The listing builds one solid part. Answer for the finished solid, in the listing's coordinates (mm). A direction names the side the tool comes from. Round coordinates to 2 decimals unless told otherwise and drop trailing zeros. Write each loop counter-clockwise with the first axis right and the second up, starting at its lowest first coordinate (ties: lowest second). Pieces come first, ordered by that corner, then holes. Notation, with made-up numbers: (13, 86) -> (58, 86) arc R21 cw to (58, 125) -> close; hole circle Ø7 at (55.25, 24.5). An arc over 180 degrees is marked (long way). Write each question's results on one line, items separated by ' | '. Start each with the question number.
```python
from build123d import *

# Parameters (mm, degrees)
SKETCH008_R           = 43
SKETCH008_R_2         = 4
PAD002_DEPTH          = 10
SKETCH009_R           = 11
POCKET002_DEPTH       = 7
SKETCH010_R           = 2.5
POCKET003_DEPTH       = 254.066565
POLARPATTERN001_COUNT = 7
SKETCH011_R           = 2.5
POCKET004_DEPTH       = 254.066565
POLARPATTERN002_COUNT = 4


with BuildPart() as sidecap:
    # Sketch008 → Pad002 (new body)
    with BuildSketch(Plane.XZ):
        Circle(SKETCH008_R)
        Circle(SKETCH008_R_2, mode=Mode.SUBTRACT)
    extrude(amount=PAD002_DEPTH)

    # Sketch009 (on Face3 of Pad002) → Pocket002 (cut)
    with BuildSketch(Plane(origin=(0, 0, 0), x_dir=(1, 0, 0), z_dir=(0, 1, 0))):
        Circle(SKETCH009_R)
    extrude(amount=-POCKET002_DEPTH, mode=Mode.SUBTRACT)

    # Sketch010 (on Face3 of Pocket002) → Pocket003 (cut, through all)
    with BuildSketch(Plane.XZ.offset(10)):
        with Locations((0, 15)):
            Circle(SKETCH010_R)
    pocket003 = extrude(amount=-POCKET003_DEPTH, mode=Mode.SUBTRACT)

    # PolarPattern001: Pocket003 ×7 about axis
    polarpattern001_axis = Axis((0, -10, 0), (0, -1, 0))
    for i in range(1, POLARPATTERN001_COUNT):
        add(pocket003.rotate(polarpattern001_axis, i * 360 / POLARPATTERN001_COUNT), mode=Mode.SUBTRACT)

    # Sketch011 (on Face3 of PolarPattern001) → Pocket004 (cut, through all)
    with BuildSketch(Plane.XZ.offset(10)):
        with Locations((0, 37.5)):
            Circle(SKETCH011_R)
    pocket004 = extrude(amount=-POCKET004_DEPTH, mode=Mode.SUBTRACT)

    # PolarPattern002: Pocket004 ×4 about axis
    polarpattern002_axis = Axis((0, -10, 0), (0, -1, 0))
    for i in range(1, POLARPATTERN002_COUNT):
        add(pocket004.rotate(polarpattern002_axis, i * 360 / POLARPATTERN002_COUNT), mode=Mode.SUBTRACT)


with BuildPart() as sidecap_1:
    # Body003 placement: moved
    add(sidecap.part.moved(Location((0, -21, 0))))


with BuildPart() as part_mirroring:
    # Part__Mirroring: instance of SideCap
    add(sidecap_1.part.mirror(Plane(origin=(0, 0, 0), x_dir=(1, 0, 0), z_dir=(0, 1, 0))))


solid = part_mirroring.part
```
Q1. Find the intervals of material crossed by line 1 (Z direction, x = 0, y = 24); line 2 (Z direction, x = 0, y = 29.3); line 3 (X direction, y = 27.5, z = 1), in increasing order.
Q2. Each of these flat-tipped pins is pushed along its axis until it touches: pin 1 (24 mm diameter, centred on x = -1, z = -3, fed in from -Y); pin 2 (2 mm diameter, centred on y = 28, z = 27, fed in from -X); pin 3 (6 mm diameter, centred on x = 29, y = 23.5, fed in from +Z); pin 4 (5 mm diameter, centred on y = 24.5, z = 16.5, fed in from -X). Where does it stop, or does it pass through?
Q3. The part is cut by section D-D, the plane z = -37.5. Write down the section's boundary in (x, y).
Q4. The part is cut by section C-C, the plane y = 23.5. State how many separate pieces and enclosed holes the cut face has, then the cut area to 3 significant figures.
Q5. For faces 1 (the cylindrical face through (-2.38, 24.45, 10.74)), 2 (the cylindrical face through (-35.06, 26.07, -0.54)), determine the directions among +Z, -Z, +X, -X, +Y, -Y from which every point of the face is accessible in a straight line to the end or side of a thin tool.
Q6. The part is cut by section B-B, the plane z = 1.5. Write down the section's boundary in (x, y).
Q7. The part is cut by section A-A, the plane x = 5.5. Write down the section's boundary in (y, z).
Answers follow:
1) line 1: -43 to -40, -35 to -11, 11 to 12.5, 17.5 to 35, 40 to 43 | line 2: -43 to -40, -35 to -4, 4 to 12.5, 17.5 to 35, 40 to 43 | line 3: -42.99 to -39.79, -35.21 to -10.95, 10.95 to 35.21, 39.79 to 42.99
2) pin 1: y = 21 | pin 2: x = -34.25 | pin 3: z = 34.25 | pin 4: x = -40.66
3) outline: (-21.04, 21) -> (-2.5, 21) -> (-2.5, 31) -> (-21.04, 31) -> close; (2.5, 21) -> (21.04, 21) -> (21.04, 31) -> (2.5, 31) -> close
4) separate pieces: 1 | enclosed holes: 12 | area: 5,210 mm^2
5) face 1: -Y | face 2: +Y, -Y
6) outline: (-42.97, 21) -> (-39.5, 21) -> (-39.5, 31) -> (-42.97, 31) -> close; (-35.5, 21) -> (-10.9, 21) -> (-10.9, 28) -> (-3.71, 28) -> (-3.71, 31) -> (-35.5, 31) -> close; (3.71, 28) -> (10.9, 28) -> (10.9, 21) -> (35.5, 21) -> (35.5, 31) -> (3.71, 31) -> close; (39.5, 21) -> (42.97, 21) -> (42.97, 31) -> (39.5, 31) -> close
7) outline: (21, -42.65) -> (31, -42.65) -> (31, -15.8) -> (21, -15.8) -> close; (21, -11.23) -> (31, -11.23) -> (31, 42.65) -> (21, 42.65) -> (21, 9.53) -> (28, 9.53) -> (28, -9.53) -> (21, -9.53) -> close
